Can you work these out from the drawing? Everything is in mm from the part's minimum corner. A direction names the side the tool comes from. Coordinates: 2 decimals unless noted, no trailing zeros. Write each loop counter-clockwise with the first axis right and the second up, starting at its lowest first coordinate (ties: lowest second). Pieces come first, ordered by that corner, then holes.
(1) Imagine slicing it at C-C, the plane z = 3.19. List the corners of the cut face in (x, y) for me.
(2) Please list where these lines run through material, in increasing order: probe 1 along X at (y, z) = (0.6, 3.19); probe 2 along X at (y, z) = (6, 5.25); probe 3 along Z at (x, y) = (22, 1).
(3) Which directions (+Z, -Z, +X, -X, +Y, -Y) give clear straight access to the entire face, cutting with the end or side of a thin tool? Please do the marked faces 4, 5, 6, 7 and 8.
(4) Imagine slicing it at A-A, the plane x = 22. List the corners of the cut face in (y, z) for me.
(5) For pin 1 Ø3 at (x, z) = (4.5, 3.5) entering from +Y; pin 2 Ø1 at (y, z) = (8, 1) entering from +X; pin 3 Ø1.9 at (y, z) = (8.5, 3) entering from -X, each with a flat end and sliding along its axis, tell me the tip position at first contact or that it passes through.
(6) Imagine slicing it at D-D, the plane x = 5.75. List the corners of the cut face in (y, z) for me.
(7) Thinking about a two-plate mould opening in Z: for the marked faces 1, 2 and 3, which applies, released by +Z, released by -Z, zero draft, split by the parting line, or undercut?
(8) Imagine slicing it at B-B, the plane y = 6.75. List the corners of the cut face in (x, z) for me, plus the area to 3 significant figures.
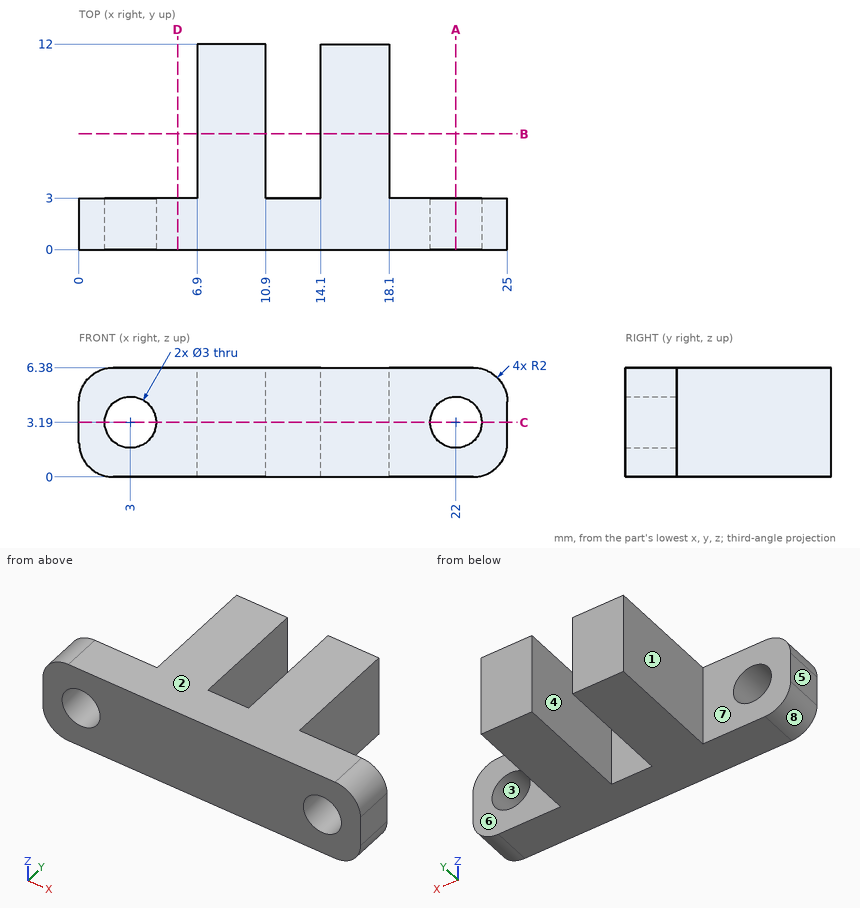
Recorded:
1. outline: (0, 0) - (1.5, 0) - (1.5, 3) - (0, 3) - close; (4.5, 0) - (20.5, 0) - (20.5, 3) - (18.1, 3) - (18.1, 12) - (14.1, 12) - (14.1, 3) - (10.9, 3) - (10.9, 12) - (6.9, 12) - (6.9, 3) - (4.5, 3) - close; (23.5, 0) - (25, 0) - (25, 3) - (23.5, 3) - close
2. probe 1: x = 0 to 1.5, 4.5 to 20.5, 23.5 to 25
2. probe 2: x = 6.9 to 10.9, 14.1 to 18.1
2. probe 3: z = 0 to 1.69, 4.69 to 6.38
3. face 4: +Z, -Z, +Y
3. face 5: +Z, -Z, -X, +Y, -Y
3. face 6: +Z, -Z, +X, +Y
3. face 7: +Z, -Z, -X, +Y
3. face 8: -Z, -X, +Y, -Y
4. outline: (0, 0) - (3, 0) - (3, 1.69) - (0, 1.69) - close; (0, 4.69) - (3, 4.69) - (3, 6.38) - (0, 6.38) - close
5. pin 1: stops at y = 3
5. pin 2: stops at x = 18.1
5. pin 3: stops at x = 6.9
6. outline: (0, 0) - (3, 0) - (3, 6.38) - (0, 6.38) - close
7. face 1: zero draft
7. face 2: released by +Z
7. face 3: undercut
8. outline: (6.9, 0) - (10.9, 0) - (10.9, 6.38) - (6.9, 6.38) - close; (14.1, 0) - (18.1, 0) - (18.1, 6.38) - (14.1, 6.38) - close
8. area: 51.0 mm2
